from build123d import *

# Parameters (mm, degrees)
SKIZZE1_R                       = 6
COMPONENT_OUTLINE_DEPTH         = 8.5
SKIZZE2_R                       = 0.5
AUFSATZ_LINEAR_AUSTRAGEN1_DEPTH = 1.7


with BuildPart() as part:
    # Skizze1 → Component_Outline (new body)
    with BuildSketch(Plane.XY):
        Circle(SKIZZE1_R)
    extrude(amount=COMPONENT_OUTLINE_DEPTH)

    # Skizze2 → Aufsatz-Linear austragen1 (add)
    with BuildSketch(Plane(origin=(0, 0, 0), x_dir=(-1, 0, 0), z_dir=(0, 0, -1))):
        with Locations(Location((-2.29, 0, 0), (0, 0, 180))):
            Circle(SKIZZE2_R)
    aufsatz_linear_austragen1 = extrude(amount=AUFSATZ_LINEAR_AUSTRAGEN1_DEPTH)

    # Spiegeln1: Aufsatz-Linear austragen1 across plane
    add(aufsatz_linear_austragen1.mirror(Plane(origin=(0, 0, 0), x_dir=(0, 0, 1), z_dir=(1, 0, 0))))


solid = part.part
Build history of the part. All positions in model axes, mm. A direction names the side the tool comes from. Coordinates: 2 decimals unless noted, no trailing zeros. Order: outer loops, then holes, each group sorted by start corner. A loop starts at its lowest first (then second) coordinate and runs counter-clockwise, first axis right, second up. Notation, with made-up numbers: (55.5, 68.25) - (92.5, 68.25) arc R15 ccw to (92.5, 96.25) - close; hole circle Ø6 at (-19.75, 60). An arc over 180 degrees is marked (long way). Write each question's results on one line, items separated by ' | '. Start each with the question number.
Item 1: Flat gauge pins, fed straight in: pin 1 (4 mm diameter, centred on y = -3, z = 4.5, fed in from +X); pin 2 (5 mm diameter, centred on x = 3, z = 2.5, fed in from -Y); pin 3 (2 mm diameter, centred on y = 4.5, z = 4, fed in from +X). Where does each tip first touch, or does it go through?
Item 2: Tool access for faces 1 (the face through (2, 0, -1.7)), 2 (the face through (2.767, -0.15, -0.838)): list every direction of +Z, -Z, +X, -X, +Y, -Y with a clear straight run to the whole face (end or side of a thin tool).
Item 3: Band-saw the part on B-B on z = -0.25. Write the cut outline in (x, y), and give its area (3 significant figures).
Item 4: Band-saw the part on D-D on z = 1. Write the cut outline in (x, y).
Item 5: Mould opens along X. For faces 3 (the face through (-6, 0, 4)), 4 (the face through (0, 0, 8.5)), 5 (the face through (-2.767, -0.15, -0.838)) say: released by +X, released by -X, zero draft, split by the parting line, or undercut.
Item 6: Band-saw the part on A-A on y = 0. Write the cut outline in (x, z), and give its area (3 significant figures).
Item 7: Band-saw the part on C-C on x = -2.29. Write the cut outline in (y, z).
Item 8: Wall check: probe 1 along Z at (x, y) = (5, 3); probe 2 along Y at (x, z) = (-5, 3); probe 3 along Y at (x, z) = (5.5, 7.5). Give the ranges that are in metal, low to high. Write a range as [from, to].
Numbers:
1) pin 1: x = 5.92 | pin 2: y = -5.98 | pin 3: x = 4.87
2) face 1: -Z, +X, -X, +Y, -Y | face 2: -Z
3) outline: circle Ø1 at (-2.29, 0); circle Ø1 at (2.29, 0) | area: 1.57 mm^2
4) outline: circle Ø12 at (0, 0)
5) face 3: split by the parting line | face 4: zero draft | face 5: undercut
6) outline: (-6, 0) - (-2.79, 0) - (-2.79, -1.7) - (-1.79, -1.7) - (-1.79, 0) - (1.79, 0) - (1.79, -1.7) - (2.79, -1.7) - (2.79, 0) - (6, 0) - (6, 8.5) - (-6, 8.5) - close | area: 105 mm^2
7) outline: (-5.55, 0) - (-0.5, 0) - (-0.5, -1.7) - (0.5, -1.7) - (0.5, 0) - (5.55, 0) - (5.55, 8.5) - (-5.55, 8.5) - close
8) probe 1: [0, 8.5] | probe 2: [-3.32, 3.32] | probe 3: [-2.4, 2.4]
